CAD build for the part. Positions are in the model's coordinates, mm. A direction names the side the tool comes from. Coordinates: 2 decimals unless noted, no trailing zeros. Loops run counter-clockwise (first coordinate to the right, second up) from the corner with the lowest first, then second, coordinate; pieces in that order, holes last. Notation, with made-up numbers: (56.5, 62) -> (73.5, 62) arc R19 cw to (73.5, 85) -> close; hole circle Ø3 at (52, 54.5). An arc over 180 degrees is marked (long way). Write each question's results on one line, items separated by ' | '.
```python
from build123d import *

# Parameters (mm, degrees)
SKETCH_1_R          = 2.5
EXTRUDE_1_DEPTH     = 55
SKETCH_2_R          = 4.25
EXTRUDE_2_DEPTH     = 5
CUT_EXTRUDE_1_DEPTH = 3
SKETCH_4_R          = 2.5
SKETCH_4_R_2        = 2
CUT_EXTRUDE_2_DEPTH = 20


with BuildPart() as part:
    # ｽｹｯﾁ1 → ﾎﾞｽ - 押し出し1 (new body)
    with BuildSketch(Plane.XY):
        Circle(SKETCH_1_R)
    extrude(amount=EXTRUDE_1_DEPTH)

    # ｽｹｯﾁ2 → ﾎﾞｽ - 押し出し2 (add)
    with BuildSketch(Plane.XY.offset(55)):
        Circle(SKETCH_2_R)
    extrude(amount=EXTRUDE_2_DEPTH)

    # ｽｹｯﾁ3 → ｶｯﾄ - 押し出し1 (cut)
    with BuildSketch(Plane.XY.offset(60)):
        Polygon((0, 2.309401077), (-2, 1.154700538), (-2, -1.154700538), (0, -2.309401077), (2, -1.154700538), (2, 1.154700538), align=None)
    extrude(amount=-CUT_EXTRUDE_1_DEPTH, mode=Mode.SUBTRACT)

    # ｽｹｯﾁ4 → ｶｯﾄ - 押し出し2 (cut)
    with BuildSketch(Plane(origin=(0, 0, 0), x_dir=(-1, 0, 0), z_dir=(0, 0, -1))):
        Circle(SKETCH_4_R)
        Circle(SKETCH_4_R_2, mode=Mode.SUBTRACT)
    extrude(amount=-CUT_EXTRUDE_2_DEPTH, mode=Mode.SUBTRACT)


solid = part.part
```
Q1. Cut at B-B on z = 9.5. Write the cut outline in (x, y), and give its area (3 significant figures).
Results are:
outline: circle Ø4 at (0, 0) | area: 12.6 mm^2
Q2. Pull direction Y, two halves, no side cores. Call faces 1 (the cylindrical face through (0, -2, 10)), 2 (the flat face through (-1.014, -1.724, 58.521)), 3 (the flat face through (1, 2, 20)): +Y half, -Y half, draft (parallel to the pull), parting line (faces both ways), or undercut.
Results are:
face 1: parting line | face 2: undercut | face 3: draft
Q3. Wall check: L1, parallel to Z at x = -4, y = -0.75; L2, parallel to Z at x = -0.5, y = -1; L3, parallel to X at y = -1.5, z = 49. Give the ranges that are in metal, low to high. Write a range as from..to.
Results are:
L1: 55..60 | L2: 0..57 | L3: -2..2
Q4. Cut at D-D on z = 37. Write the cut outline in (x, y).
Results are:
outline: circle Ø5 at (0, 0)
Q5. Which spindle directions (+Z, -Z, +X, -X, +Y, -Y) get a long thin tool onto all of the face, cutting with end or side? Do faces 4 (the flat face through (0, 0, 57)), 5 (the cylindrical face through (-0.54, -2.44, 37.25)), 6 (the flat face through (1, -2, 60)). Say none if no direction does.
Results are:
face 4: +Z | face 5: -Z | face 6: +Z, +X, -X, +Y, -Y
Q6. Cut at A-A on y = 0. Write the cut outline in (x, z), and give its area (4 significant figures).
Results are:
outline: (-4.25, 55) -> (-2.5, 55) -> (-2.5, 20) -> (-2, 20) -> (-2, 0) -> (2, 0) -> (2, 20) -> (2.5, 20) -> (2.5, 55) -> (4.25, 55) -> (4.25, 60) -> (2, 60) -> (2, 57) -> (-2, 57) -> (-2, 60) -> (-4.25, 60) -> close | area: 285.5 mm^2
Q7. Drop flat-ended pins along their axis: pin 1 (1.5 mm diameter, centred on y = 0, z = 43, fed in from +X); pin 2 (5 mm diameter, centred on x = 0, y = -2, fed in from -Z); pin 3 (3 mm diameter, centred on y = 0, z = 47.5, fed in from -X); pin 4 (3 mm diameter, centred on x = 2.5, z = 25.5, fed in from -Y). Give the stop position or say it passes through.
Results are:
pin 1: x = 2.5 | pin 2: z = 0 | pin 3: x = -2.5 | pin 4: y = -2.29
Q8. Cut at C-C on x = 0.5. Write the cut outline in (y, z).
Results are:
outline: (-4.22, 55) -> (-2.45, 55) -> (-2.45, 20) -> (-1.94, 20) -> (-1.94, 0) -> (1.94, 0) -> (1.94, 20) -> (2.45, 20) -> (2.45, 55) -> (4.22, 55) -> (4.22, 60) -> (2.02, 60) -> (2.02, 57) -> (-2.02, 57) -> (-2.02, 60) -> (-4.22, 60) -> close
